Work out the finished part from the listing and answer in its coordinate system (mm). Face numbers are marked on the shaded views. A direction names the side the tool comes from. Give positions to 0.01 mm unless a question says otherwise; leave off trailing zeros. Loops run counter-clockwise (first coordinate to the right, second up) from the corner with the lowest first, then second, coordinate; pieces in that order, holes last.
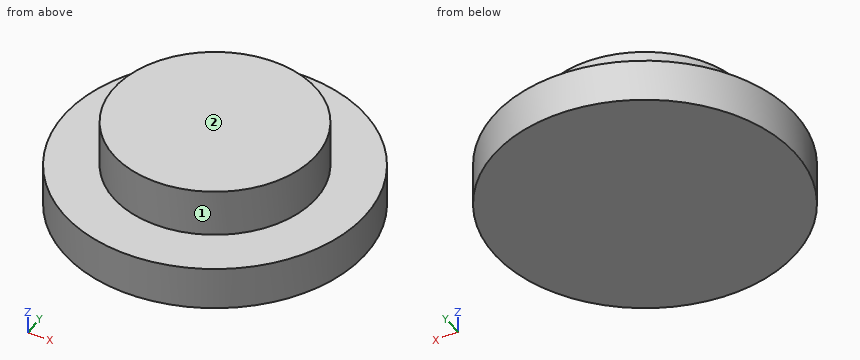
```python
from build123d import *

# Parameters (mm, degrees)
SKETCH1_R           = 4.7
BOSS_EXTRUDE1_DEPTH = 2.2
BOSS_EXTRUDE2_DEPTH = 2
SKETCH3_R           = 7
BOSS_EXTRUDE3_DEPTH = 2
SPLIT1_START        = 2.2
SPLIT1_DEPTH        = 2


# Read off the part's stored shape, not the designer's step: Split1
with BuildPart() as part:
    # Sketch1 → Boss-Extrude1 (new body)
    with BuildSketch(Plane.XY):
        Circle(SKETCH1_R)
    extrude(amount=BOSS_EXTRUDE1_DEPTH)

    # Sketch3 → Boss-Extrude3 (add)
    with BuildSketch(Plane(origin=(0, 0, 0), x_dir=(-1, 0, 0), z_dir=(0, 0, -1))):
        Circle(SKETCH3_R)
    extrude(amount=BOSS_EXTRUDE3_DEPTH)


with BuildPart() as body_2:
    # Sketch2 → Boss-Extrude2 (new body)
    with BuildSketch(Plane.XY.offset(2.2)):
        with BuildLine():
            Line((-1.76, -11.3), (-0.76, -12.3))
            Line((-0.76, -12.3), (1, -12.3))
            Line((1, -12.3), (2, -11.3))
            Line((2, -11.3), (2, -8.490583019))
            ThreePointArc((2, -8.490583019), (2.470239954, -5.460125385), (3.836734694, -2.714676203))
            ThreePointArc((3.836734694, -2.714676203), (-0.065156188, 4.699548348), (-3.76, -2.82))
            ThreePointArc((-3.76, -2.82), (-2.273167019, -5.65772234), (-1.76, -8.82))
            Line((-1.76, -8.82), (-1.76, -11.3))
        make_face()
    extrude(amount=BOSS_EXTRUDE2_DEPTH)

    # Split1 outline → Split1 (cut)
    with BuildSketch(Plane.XY.offset(SPLIT1_START)):
        with BuildLine():
            ThreePointArc((3.836734694, -2.714676203), (-0.065156188, 4.699548348), (-3.76, -2.82))
            ThreePointArc((-3.76, -2.82), (-2.273167019, -5.65772234), (-1.76, -8.82))
            Line((-1.76, -8.82), (-1.76, -11.3))
            Line((-1.76, -11.3), (-0.76, -12.3))
            Line((-0.76, -12.3), (1, -12.3))
            Line((1, -12.3), (2, -11.3))
            Line((2, -11.3), (2, -8.490583019))
            ThreePointArc((2, -8.490583019), (2.470239954, -5.460125385), (3.836734694, -2.714676203))
        make_face()
    extrude(amount=SPLIT1_DEPTH, mode=Mode.SUBTRACT)


solid = part.part
```
Q1. Which of the six approach directions +Z, -Z, +X, -X, +Y, -Y give full straight-line access (tool end or side, diameter ignored) to the marked faces 1 and 2?
Q2. Section D-D on x = 5.75 is taken. Give the vertices of the cut face in (y, z), plus the area to 3 significant figures.
Q3. Section A-A on x = 0 is taken. Give the vertices of the cut face in (y, z), plus the area to 3 significant figures.
Q4. Given pin 1 (1 mm diameter, centred on x = -2, z = 1.5, fed in from +Y); pin 2 (1.5 mm diameter, centred on y = -4.5, z = 1.5, fed in from +X); pin 3 (1.5 mm diameter, centred on x = 2.5, z = 1, fed in from +Y), each flat-ended and moving along its own axis, determine where each tip first touches the part or whether it passes through.
Q5. Section C-C on z = 0.2 is taken. Give the vertices of the cut face in (x, y), plus the area to 3 significant figures.
Q6. Consider line 1 along Z through (x, y) = (3.5, 3.75); line 2 along X through (y, z) = (3.25, -1); line 3 along X through (y, z) = (3, 1.25). Determine where each line is inside the solid, lowest interval first.
Check result:
1. face 1: +Z
1. face 2: +Z, +X, -X, +Y, -Y
2. outline: (-3.99, -2) - (3.99, -2) - (3.99, 0) - (-3.99, 0) - close
2. area: 16.0 mm2
3. outline: (-7, -2) - (7, -2) - (7, 0) - (4.7, 0) - (4.7, 2.2) - (-4.7, 2.2) - (-4.7, 0) - (-7, 0) - close
3. area: 48.7 mm2
4. pin 1: stops at y = 4.45
4. pin 2: stops at x = 2.83
4. pin 3: stops at y = 4.36
5. outline: circle Ø9.4 at (0, 0)
5. area: 69.4 mm2
6. line 1: z = -2 to 0
6. line 2: x = -6.2 to 6.2
6. line 3: x = -3.62 to 3.62
